from build123d import *

# Parameters (mm, degrees)
SKETCH_1_W                       = 78
SKETCH_1_H                       = 88
SKETCH_1_W_2                     = 70
SKETCH_1_H_2                     = 80
EXTRUDE_1_DEPTH                  = 10
SKETCH_2_W                       = 78
SKETCH_2_H                       = 88
EXTRUDE_3_DEPTH                  = 14.3
SKETCH_3_W                       = 5
SKETCH_3_H                       = 10
EXTRUDE_4_DEPTH                  = 14.3
PATTERN_LINEAR_2_COUNT           = 2
PATTERN_LINEAR_2_PITCH           = 55.4
MIRROR_3_COPY_1_SKETCH_W         = 5
MIRROR_3_COPY_1_SKETCH_H         = 10
MIRROR_3_COPY_1_DEPTH            = 14.3
SKETCH_7_W                       = 70
SKETCH_7_H                       = 80
CUT_EXTRUDE_1_DEPTH              = 10
EXTRUDE_9_DEPTH                  = 14.3
FILLET_1_R                       = 0.5
CUT_EXTRUDE_2_REACH              = 78.738
SKETCH_13_W                      = 10
SKETCH_13_H                      = 5
EXTRUDE_11_DEPTH                 = 3
SKETCH_14_R                      = 2
EXTRUDE_12_DEPTH                 = 2
SKETCH_15_R                      = 1
EXTRUDE_13_DEPTH                 = 1
PATTERN_LINEAR_3_COUNT           = 2
PATTERN_LINEAR_3_PITCH           = 65
PATTERN_LINEAR_3_COPY_1_DEPTH    = 3
PATTERN_LINEAR_3_COPY_2_SKETCH_R = 2
PATTERN_LINEAR_3_COPY_2_DEPTH    = 2
PATTERN_LINEAR_3_COPY_3_SKETCH_R = 1
PATTERN_LINEAR_3_COPY_3_DEPTH    = 1
SKETCH_16_W                      = 78
SKETCH_16_H                      = 10
EXTRUDE_14_DEPTH                 = 0.9
CUT_EXTRUDE_3_DEPTH              = 2
SKETCH_19_R                      = 0.978239546
CUT_EXTRUDE_4_DEPTH              = 77.349591778
SKETCH_20_W                      = 59.944846142
SKETCH_20_H                      = 43.194920924
CUT_EXTRUDE_5_DEPTH              = 2
FILLET_2_R                       = 3
SKETCH_23_R                      = 0.9
CUT_EXTRUDE_8_DEPTH              = 2


with BuildPart() as part:
    # 草图1 → 凸台-拉伸1 (new body)
    with BuildSketch(Plane(origin=(0, 0, 0), x_dir=(1, 0, 0), z_dir=(0, 1, 0))):
        Rectangle(SKETCH_1_W, SKETCH_1_H)
        Rectangle(SKETCH_1_W_2, SKETCH_1_H_2, mode=Mode.SUBTRACT)
    extrude(amount=EXTRUDE_1_DEPTH)

    # 草图2 → 凸台-拉伸3 (add)
    with BuildSketch(Plane.XZ):
        Rectangle(SKETCH_2_W, SKETCH_2_H)
    extrude(amount=EXTRUDE_3_DEPTH)

    # 草图3 → 凸台-拉伸4 (add)
    with BuildSketch(Plane.ZY.offset(39)):
        with Locations((41.5, 5)):
            Rectangle(SKETCH_3_W, SKETCH_3_H)
        with Locations((13, 5)):
            Rectangle(SKETCH_3_W, SKETCH_3_H)
    extrude_4 = extrude(amount=EXTRUDE_4_DEPTH)

    # 阵列(线性)2: 凸台-拉伸4 ×2
    with Locations(*[(0, 0, -i * PATTERN_LINEAR_2_PITCH) for i in range(1, PATTERN_LINEAR_2_COUNT)]):
        add(extrude_4)

    # 镜向3: 凸台-拉伸4 across plane
    add(extrude_4.mirror(Plane(origin=(0, 0, 0), x_dir=(0, 0, 1), z_dir=(1, 0, 0))))

    # 镜向3 copy 1 sketch → 镜向3 copy 1 (add)
    with BuildSketch(Plane(origin=(39, 0, -55.4), x_dir=(0, 0, 1), z_dir=(1, 0, 0))):
        with Locations((41.5, -5)):
            Rectangle(MIRROR_3_COPY_1_SKETCH_W, MIRROR_3_COPY_1_SKETCH_H)
        with Locations((13, -5)):
            Rectangle(MIRROR_3_COPY_1_SKETCH_W, MIRROR_3_COPY_1_SKETCH_H)
    extrude(amount=MIRROR_3_COPY_1_DEPTH)

    # 草图7 → 切除-拉伸1 (cut)
    with BuildSketch(Plane(origin=(0, 0, 0), x_dir=(1, 0, 0), z_dir=(0, 1, 0))):
        Rectangle(SKETCH_7_W, SKETCH_7_H)
    extrude(amount=-CUT_EXTRUDE_1_DEPTH, mode=Mode.SUBTRACT)

    # 草图12 → 凸台-拉伸9 (add)
    with BuildSketch(Plane.XZ.offset(14.3)):
        Polygon((-39, -44), (0, -49.570884246), (39, -44), align=None)
    extrude(amount=-EXTRUDE_9_DEPTH)

    # 圆角1
    fillet_1_edges = [part.edges().sort_by_distance(p)[0] for p in [
        (53.3, 5, 15.5),
        (53.3, 5, 10.5),
        (53.3, 5, -11.4),
        (53.3, 5, -16.4),
        (53.3, 5, -39.9),
        (53.3, 5, -44.9),
        (-53.3, 5, 44),
        (-53.3, 5, 39),
        (-53.3, 5, 15.5),
        (-53.3, 5, 10.5),
        (-53.3, 5, -11.4),
        (-53.3, 5, -16.4),
        (-53.3, 5, -39.9),
        (-53.3, 5, -44.9),
        (53.3, 5, 44),
        (53.3, 5, 39),
    ]]
    fillet(fillet_1_edges, radius=FILLET_1_R)

    # 草图13 → 切除-拉伸2 (cut, up to next)
    with BuildSketch(Plane.XZ.offset(14.3), mode=Mode.PRIVATE) as cut_extrude_2_sk1:
        with Locations((-28, -34.5)):
            Rectangle(SKETCH_13_W, SKETCH_13_H)
    cut_extrude_2_tool1 = extrude(cut_extrude_2_sk1.sketch, amount=-CUT_EXTRUDE_2_REACH, mode=Mode.PRIVATE) & part.part
    # 草图13 → 切除-拉伸2 (cut, up to next)
    with BuildSketch(Plane.XZ.offset(14.3), mode=Mode.PRIVATE) as cut_extrude_2_sk2:
        with Locations((-28, 16.5)):
            Rectangle(SKETCH_13_W, SKETCH_13_H)
    cut_extrude_2_tool2 = extrude(cut_extrude_2_sk2.sketch, amount=-CUT_EXTRUDE_2_REACH, mode=Mode.PRIVATE) & part.part
    # 草图13 → 切除-拉伸2 (cut, up to next)
    with BuildSketch(Plane.XZ.offset(14.3), mode=Mode.PRIVATE) as cut_extrude_2_sk3:
        with Locations((28, -34.5)):
            Rectangle(SKETCH_13_W, SKETCH_13_H)
    cut_extrude_2_tool3 = extrude(cut_extrude_2_sk3.sketch, amount=-CUT_EXTRUDE_2_REACH, mode=Mode.PRIVATE) & part.part
    # 草图13 → 切除-拉伸2 (cut, up to next)
    with BuildSketch(Plane.XZ.offset(14.3), mode=Mode.PRIVATE) as cut_extrude_2_sk4:
        with Locations((28, 16.5)):
            Rectangle(SKETCH_13_W, SKETCH_13_H)
    cut_extrude_2_tool4 = extrude(cut_extrude_2_sk4.sketch, amount=-CUT_EXTRUDE_2_REACH, mode=Mode.PRIVATE) & part.part
    add(cut_extrude_2_tool1.solids().sort_by_distance((-28, -14.3, -34.5))[0], mode=Mode.SUBTRACT)
    add(cut_extrude_2_tool2.solids().sort_by_distance((-28, -14.3, 16.5))[0], mode=Mode.SUBTRACT)
    add(cut_extrude_2_tool3.solids().sort_by_distance((28, -14.3, -34.5))[0], mode=Mode.SUBTRACT)
    add(cut_extrude_2_tool4.solids().sort_by_distance((28, -14.3, 16.5))[0], mode=Mode.SUBTRACT)

    # 草图8 → 凸台-拉伸11 (add)
    with BuildSketch(Plane.XZ.offset(14.3)):
        with BuildLine():
            Line((47.25, -26.060000002), (39, -26.060000002))
            Line((39, -26.060000002), (39, -38.559799845))
            Line((39, -38.559799845), (39, -39.039999998))
            Line((39, -39.039999998), (47.25, -39.039999998))
            ThreePointArc((47.25, -39.039999998), (53.739999998, -32.55), (47.25, -26.060000002))
        make_face()
    extrude_11 = extrude(amount=-EXTRUDE_11_DEPTH)

    # 草图14 → 凸台-拉伸12 (add)
    with BuildSketch(Plane(origin=(0, -11.3, 0), x_dir=(1, 0, 0), z_dir=(0, 1, 0))):
        with Locations(Location((47.25, 32.55, 0), (0, 0, 90))):
            Circle(SKETCH_14_R)
    extrude_12 = extrude(amount=EXTRUDE_12_DEPTH)

    # 草图15 → 凸台-拉伸13 (add)
    with BuildSketch(Plane(origin=(0, -9.3, 0), x_dir=(1, 0, 0), z_dir=(0, 1, 0))):
        with Locations(Location((47.25, 32.55, 0), (0, 0, 270))):
            Circle(SKETCH_15_R)
    extrude_13 = extrude(amount=EXTRUDE_13_DEPTH)

    # 镜向4: 凸台-拉伸11, 凸台-拉伸12, 凸台-拉伸13 across plane
    add(extrude_11.mirror(Plane(origin=(0, 0, 0), x_dir=(0, 0, 1), z_dir=(1, 0, 0))))
    add(extrude_12.mirror(Plane(origin=(0, 0, 0), x_dir=(0, 0, 1), z_dir=(1, 0, 0))))
    add(extrude_13.mirror(Plane(origin=(0, 0, 0), x_dir=(0, 0, 1), z_dir=(1, 0, 0))))

    # 阵列(线性)3: 凸台-拉伸11, 凸台-拉伸12, 凸台-拉伸13 ×2
    with Locations(*[(0, 0, i * PATTERN_LINEAR_3_PITCH) for i in range(1, PATTERN_LINEAR_3_COUNT)]):
        add(extrude_11)
        add(extrude_12)
        add(extrude_13)

    # 阵列(线性)3 copy 1 sketch → 阵列(线性)3 copy 1 (add)
    with BuildSketch(Plane(origin=(0, -14.3, 65), x_dir=(-1, 0, 0), z_dir=(0, -1, 0))):
        with BuildLine():
            Line((47.25, 26.060000002), (39, 26.060000002))
            Line((39, 26.060000002), (39, 38.559799845))
            Line((39, 38.559799845), (39, 39.039999998))
            Line((39, 39.039999998), (47.25, 39.039999998))
            ThreePointArc((47.25, 39.039999998), (53.739999998, 32.55), (47.25, 26.060000002))
        make_face()
    extrude(amount=-PATTERN_LINEAR_3_COPY_1_DEPTH)

    # 阵列(线性)3 copy 2 sketch → 阵列(线性)3 copy 2 (add)
    with BuildSketch(Plane(origin=(0, -11.3, 65), x_dir=(-1, 0, 0), z_dir=(0, 1, 0))):
        with Locations((47.25, -32.55)):
            Circle(PATTERN_LINEAR_3_COPY_2_SKETCH_R)
    extrude(amount=PATTERN_LINEAR_3_COPY_2_DEPTH)

    # 阵列(线性)3 copy 3 sketch → 阵列(线性)3 copy 3 (add)
    with BuildSketch(Plane(origin=(0, -9.3, 65), x_dir=(-1, 0, 0), z_dir=(0, 1, 0))):
        with Locations((47.25, -32.55)):
            Circle(PATTERN_LINEAR_3_COPY_3_SKETCH_R)
    extrude(amount=PATTERN_LINEAR_3_COPY_3_DEPTH)

    # 草图16 → 凸台-拉伸14 (add)
    with BuildSketch(Plane(origin=(0, 0, -44), x_dir=(-1, 0, 0), z_dir=(0, 0, -1))):
        with Locations((0, 5)):
            Rectangle(SKETCH_16_W, SKETCH_16_H)
    extrude(amount=EXTRUDE_14_DEPTH)

    # 草图18 → 切除-拉伸3 (cut)
    with BuildSketch(Plane(origin=(0, -10, 0), x_dir=(1, 0, 0), z_dir=(0, 1, 0))):
        with BuildLine():
            Line((-31.5, 28), (-31.5, -10))
            ThreePointArc((-31.5, -10), (-30.914213562, -11.414213562), (-29.5, -12))
            Line((-29.5, -12), (24.5, -12))
            ThreePointArc((24.5, -12), (25.914213562, -11.414213562), (26.5, -10))
            Line((26.5, -10), (26.5, 28))
            ThreePointArc((26.5, 28), (25.914213562, 29.414213562), (24.5, 30))
            Line((24.5, 30), (-29.5, 30))
            ThreePointArc((-29.5, 30), (-30.914213562, 29.414213562), (-31.5, 28))
        make_face()
    extrude(amount=-CUT_EXTRUDE_3_DEPTH, mode=Mode.SUBTRACT)

    # 草图19 → 切除-拉伸4 (cut, through all)
    with BuildSketch(Plane(origin=(0, -12, 0), x_dir=(1, 0, 0), z_dir=(0, 1, 0))):
        with Locations(Location((22.5, 26, 0), (0, 0, 270))):
            Circle(SKETCH_19_R)
        with Locations(Location((22.5, -8, 0), (0, 0, 270))):
            Circle(SKETCH_19_R)
        with Locations(Location((-27.5, -8, 0), (0, 0, 270))):
            Circle(SKETCH_19_R)
        with Locations(Location((-27.5, 26, 0), (0, 0, 270))):
            Circle(SKETCH_19_R)
    extrude(amount=-CUT_EXTRUDE_4_DEPTH, mode=Mode.SUBTRACT)

    # 草图20 → 切除-拉伸5 (cut)
    with BuildSketch(Plane(origin=(0, -12, 0), x_dir=(1, 0, 0), z_dir=(0, 1, 0))):
        with Locations((-2.5, 9)):
            Rectangle(SKETCH_20_W, SKETCH_20_H)
    extrude(amount=CUT_EXTRUDE_5_DEPTH, mode=Mode.SUBTRACT)

    # 圆角2
    fillet_2_edges = [part.edges().sort_by_distance(p)[0] for p in [
        (39, -12.8, -39.039999998),
        (39, -12.8, -26.060000002),
        (-39, -12.8, -26.060000002),
        (-39, -12.8, -39.039999998),
        (-39, -12.8, 38.939999998),
        (-39, -12.8, 25.960000002),
    ]]
    fillet(fillet_2_edges, radius=FILLET_2_R)

    # 草图23 → 切除-拉伸8 (cut)
    with BuildSketch(Plane(origin=(0, 10, 0), x_dir=(1, 0, 0), z_dir=(0, 1, 0))):
        with Locations(Location((-47.25, -41.122009123, 0), (0, 0, 270))):
            Circle(SKETCH_23_R)
        with Locations(Location((-47.25, -13.877990877, 0), (0, 0, 270))):
            Circle(SKETCH_23_R)
        with Locations(Location((-47.25, 13.977990877, 0), (0, 0, 270))):
            Circle(SKETCH_23_R)
        with Locations(Location((-47.25, 41.222009123, 0), (0, 0, 270))):
            Circle(SKETCH_23_R)
        with Locations(Location((47.25, -41.122009123, 0), (0, 0, 270))):
            Circle(SKETCH_23_R)
        with Locations(Location((47.25, -13.877990877, 0), (0, 0, 270))):
            Circle(SKETCH_23_R)
        with Locations(Location((47.25, 13.977990877, 0), (0, 0, 270))):
            Circle(SKETCH_23_R)
        with Locations(Location((47.25, 41.222009123, 0), (0, 0, 270))):
            Circle(SKETCH_23_R)
    extrude(amount=-CUT_EXTRUDE_8_DEPTH, mode=Mode.SUBTRACT)


solid = part.part
The model under review builds one solid part; all positions refer to its coordinate system, in mm. A direction names the side the tool comes from. Coordinates: 2 decimals unless noted, no trailing zeros. Loops run counter-clockwise (first coordinate to the right, second up) from the corner with the lowest first, then second, coordinate; pieces in that order, holes last. Notation, with made-up numbers: (-10.75, 46.5) -> (7.25, 46.5) arc R26 cw to (7.25, 68.5) -> close; hole circle Ø2 at (-3, -13). An arc over 180 degrees is marked (long way). Use a Markdown table: item, result. Add a question column.
1. Machinability: for faces 1 (the face through (35, 0, 1)), 2 (the face through (-23, -12, 16)), 3 (the face through (0, 0, -47)), 4 (the face through (-45, -13, -26.06)), 5 (the face through (-39.9, -12.8, -39.9)), which of the approach directions +Z, -Z, +X, -X, +Y, -Y give a long, thin tool a straight path to every point of the face, cutting with its end or side? Answer none if there is none.
2. Add section C-C on x = 4. Write out the cut boundary in (y, z).
3. To check wall thickness, follow line 1 (Z direction, x = 49, y = 2.25); line 2 (X direction, y = 7, z = 19.5); line 3 (Y direction, x = -8.5, z = -11). State the ranges of each line that lie inside material, in increasing order.
4. Draft analysis for pull direction Z (two halves, no side actions). For faces 6 (the face through (43, -13, 38.94)), 7 (the face through (-33, -12, -35)), 8 (the face through (-45, 0, -42)), state which applies: pulls with the +Z half, pulls with the -Z half, needs draft (parallel to the pull), parting line crosses it, or undercut.
5. Add section A-A on x = -25. Write out the cut boundary in (y, z).
6. Clearance check with flat-ended pins moving along their axes: pin 1 Ø0.6 at (y, z) = (-10.5, -8.5) entering from +X; pin 2 Ø4 at (y, z) = (-7.5, -13) entering from -X; pin 3 Ø4.5 at (y, z) = (2.5, 12.5) entering from +X. State where each tip first meets the part, or that it passes through.
7. Add section B-B on z = -10. Write out the cut boundary in (x, y).
Returned:
| question | item | result |
|---|---|---|
| 1 | face 1 | +Y |
| 1 | face 2 | +Y, -Y |
| 1 | face 3 | -Z, +X, -X, +Y |
| 1 | face 4 | -X, +Y, -Y |
| 1 | face 5 | -Z, -X, -Y |
| 2 | outline | (-14.3, -49) -> (0, -49) -> (0, -44.9) -> (10, -44.9) -> (10, -40) -> (-10, -40) -> (-10, -30.6) -> (-12, -30.6) -> (-12, 12.6) -> (-10, 12.6) -> (-10, 40) -> (10, 40) -> (10, 44) -> (-14.3, 44) -> close |
| 3 | line 1 | z = -44.9 to -39.9, -16.4 to -11.4, 10.5 to 15.5, 39 to 44 |
| 3 | line 2 | x = -39 to -35, 35 to 39 |
| 3 | line 3 | y = -14.3 to -12 |
| 4 | face 6 | pulls with the +Z half |
| 4 | face 7 | undercut |
| 4 | face 8 | needs draft |
| 5 | outline | (-14.3, -46) -> (0, -46) -> (0, -44.9) -> (10, -44.9) -> (10, -40) -> (-10, -40) -> (-10, -37) -> (-14.3, -37) -> close; (-14.3, -32) -> (-10, -32) -> (-10, -30.6) -> (-12, -30.6) -> (-12, 12.6) -> (-10, 12.6) -> (-10, 14) -> (-14.3, 14) -> close; (-14.3, 19) -> (-10, 19) -> (-10, 40) -> (10, 40) -> (10, 44) -> (-14.3, 44) -> close |
| 6 | pin 1 | stops at x = 39 |
| 6 | pin 2 | stops at x = -39 |
| 6 | pin 3 | stops at x = 53.3 |
| 7 | outline | (-39, -14.3) -> (39, -14.3) -> (39, 10) -> (35, 10) -> (35, -10) -> (27.47, -10) -> (27.47, -12) -> (-32.47, -12) -> (-32.47, -10) -> (-35, -10) -> (-35, 10) -> (-39, 10) -> close |
